from build123d import *

# Parameters (mm, degrees)
SKETCH_1_W          = 126.2
SKETCH_1_H          = 156
EXTRUDE_1_DEPTH     = 31
CUT_EXTRUDE_START   = -26
CUT_EXTRUDE_1_DEPTH = 26
FILLET_1_R          = 5
F_12_0MM_1_D        = 12
F_12_0MM_1_DEPTH    = 17
F_12_0MM_1_TIP      = 3.605163714
SKETCH_6_R          = 2.1
CUT_EXTRUDE_2_DEPTH = 10
SKETCH_7_R          = 2.1
CUT_EXTRUDE_3_DEPTH = 10
CHAMFER_1_SIZE      = 3


with BuildPart() as part:
    # 草图1 → 凸台-拉伸1 (new body)
    with BuildSketch(Plane(origin=(0, 0, 0), x_dir=(1, 0, 0), z_dir=(0, 1, 0))):
        with Locations((-4.2, 0)):
            Rectangle(SKETCH_1_W, SKETCH_1_H)
        with BuildLine():
            Line((-42.5, 75.1), (42.5, 75.1))
            ThreePointArc((42.5, 75.1), (48.995331881, 71.581118318), (51.1, 64.5))
            Line((51.1, 64.5), (51.1, -64.5))
            ThreePointArc((51.1, -64.5), (48.995331881, -71.581118318), (42.5, -75.1))
            Line((42.5, -75.1), (-42.5, -75.1))
            ThreePointArc((-42.5, -75.1), (-48.995331881, -71.581118318), (-51.1, -64.5))
            Line((-51.1, -64.5), (-51.1, 64.5))
            ThreePointArc((-51.1, 64.5), (-48.995331881, 71.581118318), (-42.5, 75.1))
        make_face(mode=Mode.SUBTRACT)
    extrude(amount=EXTRUDE_1_DEPTH)

    # 草图2 → 切除-拉伸1 (cut)
    with BuildSketch(Plane(origin=(0, 31, 0), x_dir=(1, 0, 0), z_dir=(0, 1, 0)).offset(CUT_EXTRUDE_START)):
        with BuildLine():
            Line((-42.780928277, -74.780928277), (-43.029918625, -75.029918625))
            ThreePointArc((-43.029918625, -75.029918625), (-42.765444551, -75.068628433), (-42.5, -75.1))
            Line((-42.5, -75.1), (-42.780928277, -74.780928277))
        make_face()
        with BuildLine():
            Line((-43.029918625, -75.029918625), (-43.1, -75.1))
            Line((-43.1, -75.1), (-42.5, -75.1))
            ThreePointArc((-42.5, -75.1), (-42.765444551, -75.068628433), (-43.029918625, -75.029918625))
        make_face()
        Polygon((43.1, -75.1), (42.5, -75.1), (-42.5, -75.1), (-43.1, -75.1), (-46, -78), (46, -78), align=None)
        with BuildLine():
            ThreePointArc((42.5, -75.1), (42.765444551, -75.068628433), (43.029918625, -75.029918625))
            Line((43.029918625, -75.029918625), (42.872377268, -74.872377268))
            Line((42.872377268, -74.872377268), (42.5, -75.1))
        make_face()
        with BuildLine():
            Line((42.5, -75.1), (43.1, -75.1))
            Line((43.1, -75.1), (43.029918625, -75.029918625))
            ThreePointArc((43.029918625, -75.029918625), (42.765444551, -75.068628433), (42.5, -75.1))
        make_face()
        Polygon((46, 78), (-46, 78), (-43.1, 75.1), (-42.5, 75.1), (42.5, 75.1), (43.1, 75.1), align=None)
        with BuildLine():
            Line((-42.780928277, 74.780928277), (-42.5, 75.1))
            ThreePointArc((-42.5, 75.1), (-42.765444551, 75.068628433), (-43.029918625, 75.029918625))
            Line((-43.029918625, 75.029918625), (-42.780928277, 74.780928277))
        make_face()
        with BuildLine():
            Line((-42.5, 75.1), (-43.1, 75.1))
            Line((-43.1, 75.1), (-43.029918625, 75.029918625))
            ThreePointArc((-43.029918625, 75.029918625), (-42.765444551, 75.068628433), (-42.5, 75.1))
        make_face()
        with BuildLine():
            ThreePointArc((43.029918625, 75.029918625), (42.765444551, 75.068628433), (42.5, 75.1))
            Line((42.5, 75.1), (42.872377268, 74.872377268))
            Line((42.872377268, 74.872377268), (43.029918625, 75.029918625))
        make_face()
        with BuildLine():
            Line((43.029918625, 75.029918625), (43.1, 75.1))
            Line((43.1, 75.1), (42.5, 75.1))
            ThreePointArc((42.5, 75.1), (42.765444551, 75.068628433), (43.029918625, 75.029918625))
        make_face()
    extrude(amount=CUT_EXTRUDE_1_DEPTH, mode=Mode.SUBTRACT)

    # 圆角1
    fillet_1_edges = [part.edges().sort_by_distance(p)[0] for p in [
        (58.9, 15.5, -78),
        (58.9, 15.5, 78),
        (-67.3, 15.5, 78),
        (-67.3, 15.5, -78),
    ]]
    fillet(fillet_1_edges, radius=FILLET_1_R)

    # Ø12.0mm 暗销孔1
    with Locations(Plane(origin=(58.9, 0, 0), x_dir=(0, 0, -1), z_dir=(1, 0, 0))):
        with Locations((42, 19.55), (-42, 19.55)):
            Hole(F_12_0MM_1_D / 2, depth=F_12_0MM_1_DEPTH)
            with Locations((0, 0, -(F_12_0MM_1_DEPTH + F_12_0MM_1_TIP / 2))):  # 118° drill point
                Cone(0, F_12_0MM_1_D / 2, F_12_0MM_1_TIP, mode=Mode.SUBTRACT)

    # 草图6 → 切除-拉伸2 (cut)
    with BuildSketch(Plane.ZY.offset(67.3)):
        with Locations((-11, 13.95)):
            Circle(SKETCH_6_R)
        with Locations(Location((11, 13.95, 0), (0, 0, 180))):
            Circle(SKETCH_6_R)
    extrude(amount=-CUT_EXTRUDE_2_DEPTH, mode=Mode.SUBTRACT)

    # 草图7 → 切除-拉伸3 (cut)
    with BuildSketch(Plane.XZ):
        with Locations(Location((-58.493442579, 70.964337058, 0), (0, 0, 270))):
            Circle(SKETCH_7_R)
        with Locations(Location((53.705008218, 73.348219362, 0), (0, 0, 270))):
            Circle(SKETCH_7_R)
        with Locations(Location((-58.493442579, -70.964337058, 0), (0, 0, 270))):
            Circle(SKETCH_7_R)
        with Locations(Location((53.705008218, -73.348219362, 0), (0, 0, 270))):
            Circle(SKETCH_7_R)
    extrude(amount=-CUT_EXTRUDE_3_DEPTH, mode=Mode.SUBTRACT)

    # 倒角1
    chamfer_1_edges = [part.edges().sort_by_distance(p)[0] for p in [
        (58.9, 19.55, 36),
        (58.9, 19.55, -48),
    ]]
    chamfer(chamfer_1_edges, length=CHAMFER_1_SIZE)


solid = part.part
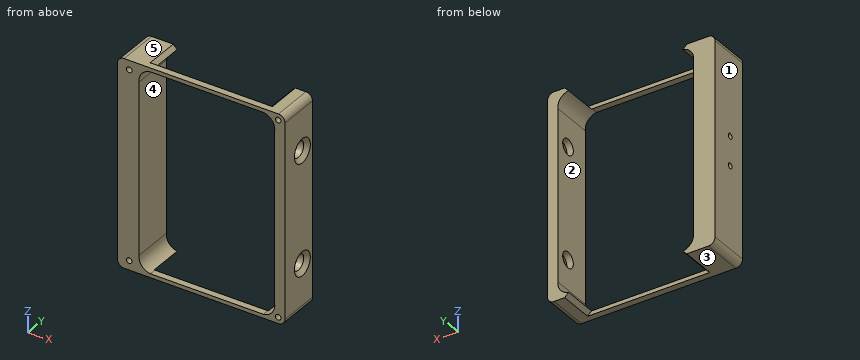
Could you check a few things on this model? Use its own coordinates, in mm. Face numbers are marked on the shaded views. A direction names the side the tool comes from. Give positions to 0.01 mm unless a question says otherwise; leave off trailing zeros. Write each loop counter-clockwise with the first axis right and the second up, starting at its lowest first coordinate (ties: lowest second). Pieces come first, ordered by that corner, then holes. Notation, with made-up numbers: (48.5, 46.25) - (68.5, 46.25) arc R16 cw to (68.5, 58.25) - close; hole circle Ø8 at (19.25, 39.5). An arc over 180 degrees is marked (long way). Use CSV: the item, a comma, the result in double quotes. Start each with the question number.
Item 1: I want a section at C-C, the plane z = -42. Please give me the cut outline in (x, y).
Item 2: If I drill on line 1 along X through (y, z) = (7, 31); line 2 along X through (y, z) = (14, -65.5); line 3 along X through (y, z) = (7.5, 71), over which ranges is the centre line in solid material (lowest first)?
Item 3: I'm going to push flat-ended pins straight in: pin 1 (4 mm diameter, centred on y = 13.95, z = 11, fed in from -X); pin 2 (11 mm diameter, centred on y = 19.55, z = -42, fed in from +X); pin 3 (3.5 mm diameter, centred on x = -15.5, z = 76.5, fed in from +Y). Where does each tip first touch, or does it pass through?
Item 4: I want a section at A-A, the plane x = -21. Please give me the cut outline in (y, z).
Item 5: I want a section at B-B, the plane z = -11. Please give me the cut outline in (x, y), then the cut area to 3 significant figures.
Item 6: For the marked faces 4 and 5, which set-ups out of +Z, -Z, +X, -X, +Y, -Y let a thin tool reach every point of the face, with its end or its side?
Item 7: If we mould it in two halves opening along X, with no side actions, what happens to the marked faces 1, 2 and 3? For each: pulls with the +X half, pulls with the -X half, needs draft (parallel to the pull), parting line crosses it, or undercut.
Findings:
1,outline,"(-67.3, 0) - (-51.1, 0) - (-51.1, 31) - (-67.3, 31) - close; (51.1, 0) - (58.9, 0) - (58.9, 10.55) - (55.9, 13.55) - (51.1, 13.55) - close; (51.1, 25.55) - (55.9, 25.55) - (58.9, 28.55) - (58.9, 31) - (51.1, 31) - close"
2,line 1,"x = -67.3 to -51.1, 51.1 to 58.9"
2,line 2,"x = -67.3 to -51.15, 51.15 to 58.9"
2,line 3,"x = -67.3 to -60.59, -56.39 to -49.43, 49.43 to 58.9"
3,pin 1,"stops at x = -57.3"
3,pin 2,"stops at x = -51.1"
3,pin 3,"stops at y = 5"
4,outline,"(0, -78) - (5, -78) - (5, -75.1) - (0, -75.1) - close; (0, 75.1) - (5, 75.1) - (5, 78) - (0, 78) - close"
5,outline,"(-67.3, 0) - (-51.1, 0) - (-51.1, 31) - (-67.3, 31) - (-67.3, 16.05) - (-57.3, 16.05) - (-57.3, 11.85) - (-67.3, 11.85) - close; (51.1, 0) - (58.9, 0) - (58.9, 31) - (51.1, 31) - close"
5,area,"702 mm2"
6,face 4,"+Y, -Y"
6,face 5,"+Z, +X, -X, +Y, -Y"
7,face 1,"pulls with the -X half"
7,face 2,"undercut"
7,face 3,"needs draft"
